```python
from build123d import *

# Parameters (mm, degrees)
F1_DEPTH = 16.51
F2_DEPTH = 5.08


with BuildPart() as f1:
    # F0 (on Right) → F1 (new body)
    with BuildSketch(Plane.YZ):
        Polygon((-10.969255, -8.832134), (-16.518005, -8.832134), (-16.518005, -12.155996), (15.231995, -12.41384), (15.231995, -8.832134), (7.611995, -8.832134), align=None)
    extrude(amount=F1_DEPTH)

    # F0 (on Right) → F2 (join)
    with BuildSketch(Plane.YZ):
        Polygon((-5.86939, 20.09064), (-7.352562, 11.67915), (7.611995, -8.832134), (15.231995, -8.832134), align=None)
        Polygon((-5.050279, 56.20457), (-16.518005, -8.832134), (-10.969255, -8.832134), (-7.352562, 11.67915), (-5.86939, 20.09064), (0.498471, 56.20457), align=None)
    extrude(amount=F2_DEPTH)

    # F3: F1 across face


with BuildPart() as f1_1:
    add(f1.part)
    add(f1.part.mirror(Plane(origin=(16.51, -0.445421, -10.559328), x_dir=(0, 1, 0), z_dir=(1, 0, 0))))


solid = f1_1.part
```
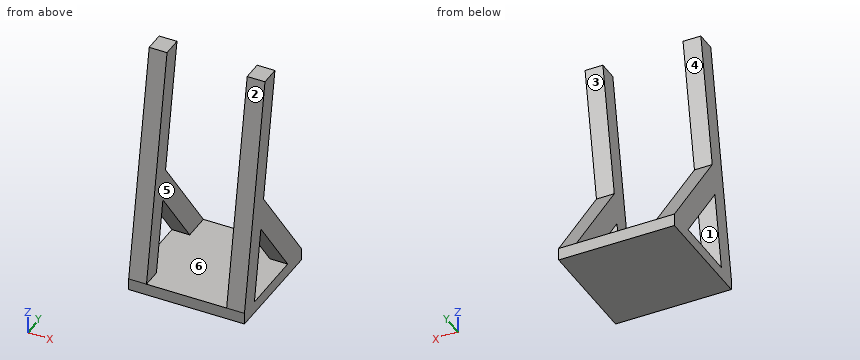
Read the model definition and answer for the solid it produces. Units are mm, in the model's axes. Face numbers are marked on the shaded views. A direction names the side the tool comes from. Coordinates: 2 decimals unless noted, no trailing zeros. Write each loop counter-clockwise with the first axis right and the second up, starting at its lowest first coordinate (ties: lowest second). Pieces come first, ordered by that corner, then holes. Notation, with made-up numbers: (73.25, 11.5) -> (115.25, 11.5) arc R13 cw to (115.25, 27.5) -> close; hole circle Ø7 at (86.25, 45). An arc over 180 degrees is marked (long way). Write item = value, one per line.
(1) Section D-D on z = 25.5 is taken. Write down the section's boundary in (x, y), plus the area to 3 significant figures.
From the geometry:
outline = (0, -10.46) -> (5.08, -10.46) -> (5.08, -4.92) -> (0, -4.92) -> close; (27.94, -10.46) -> (33.02, -10.46) -> (33.02, -4.92) -> (27.94, -4.92) -> close
area = 56.4 mm2
(2) Section C-C on x = 29.5 is taken. Write down the section's boundary in (y, z).
From the geometry:
outline = (-16.52, -12.16) -> (15.23, -12.41) -> (15.23, -8.83) -> (-5.87, 20.09) -> (0.5, 56.2) -> (-5.05, 56.2) -> (-16.52, -8.83) -> close; hole (-10.97, -8.83) -> (7.61, -8.83) -> (-7.35, 11.68) -> close
(3) Section B-B on z = -1.5 is taken. Write down the section's boundary in (x, y), plus the area to 3 significant figures.
From the geometry:
outline = (0, -15.23) -> (5.08, -15.23) -> (5.08, -9.68) -> (0, -9.68) -> close; (0, 2.26) -> (5.08, 2.26) -> (5.08, 9.88) -> (0, 9.88) -> close; (27.94, -15.23) -> (33.02, -15.23) -> (33.02, -9.68) -> (27.94, -9.68) -> close; (27.94, 2.26) -> (33.02, 2.26) -> (33.02, 9.88) -> (27.94, 9.88) -> close
area = 134 mm2
(4) Given pin 1 Ø5 at (x, y) = (16, 2) entering from +Z; pin 2 Ø10 at (x, y) = (5, -9.5) entering from -Z; pin 3 Ø3 at (x, y) = (8.5, -9) entering from -Z, each flat-ended and moving along its own axis, determine where each tip first touches the part or whether it passes through.
From the geometry:
pin_1 = -8.83
pin_2 = -12.25
pin_3 = -12.23
(5) Section A-A on y = -10 is taken. Write down the section's boundary in (x, z).
From the geometry:
outline = (0, -12.21) -> (33.02, -12.21) -> (33.02, -8.83) -> (0, -8.83) -> close; (0, -3.34) -> (5.08, -3.34) -> (5.08, 28.13) -> (0, 28.13) -> close; (27.94, -3.34) -> (33.02, -3.34) -> (33.02, 28.13) -> (27.94, 28.13) -> close
(6) For a pull along Y with two mould halves and no side action, classify the marked faces 1, 2 and 3 as +Y half, -Y half, draft (parallel to the pull), parting line (faces both ways), or undercut.
From the geometry:
face_1 = undercut
face_2 = -Y half
face_3 = +Y half
(7) Straight lines are drawn through the part: L1, parallel to X at y = 10.5, z = -8; L2, parallel to Z at x = 4.5, y = 3; L3, parallel to Z at x = 11, y = -15. For each, find the intervals that lie inside material, in ascending order. Write a range as from..to.
From the geometry:
L1 = 0..5.08, 27.94..33.02
L2 = -12.31..-8.83, -2.51..7.93
L3 = -12.17..-8.83
(8) Which of the six approach directions +Z, -Z, +X, -X, +Y, -Y give full straight-line access (tool end or side, diameter ignored) to the marked faces 4, 5 and 6?
From the geometry:
face_4 = +X, -X, +Y
face_5 = +Z, +Y, -Y
face_6 = none
